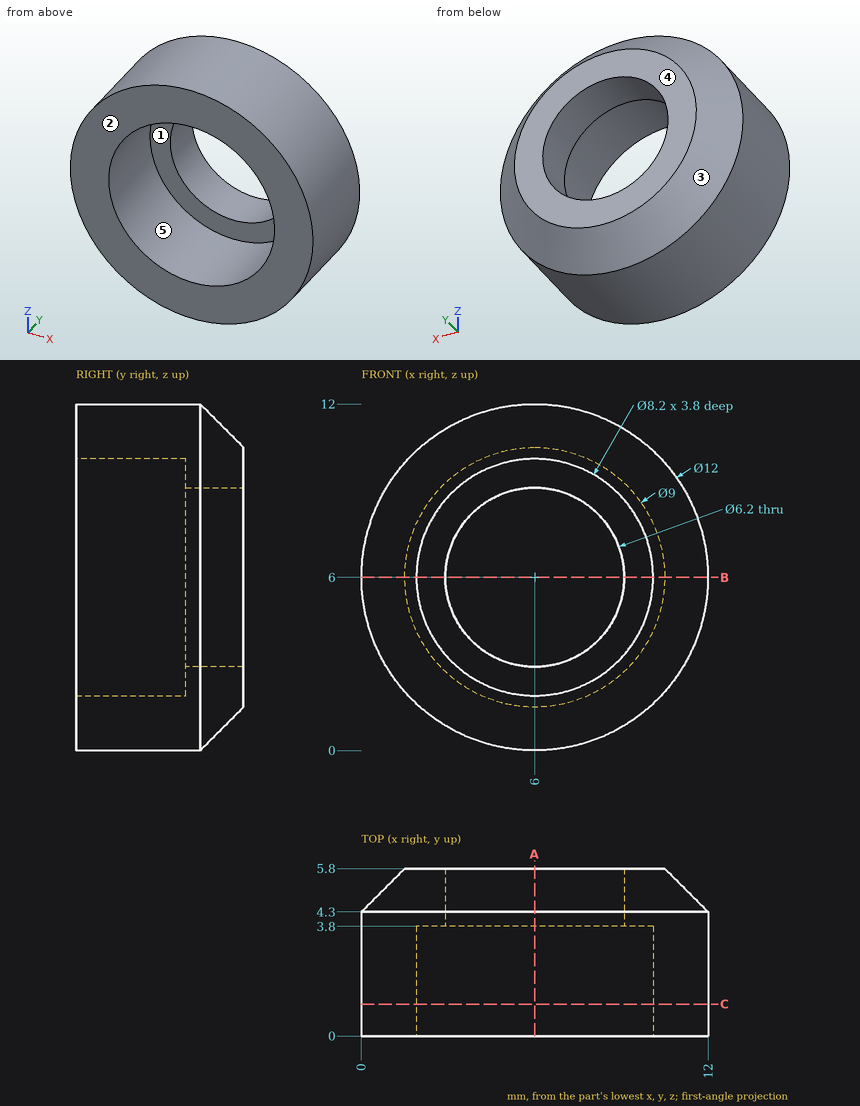
The drawing under review shows one solid part. Ordinate dimensions are in mm from its lowest x, y, z. A direction names the side the tool comes from. Round coordinates to 2 decimals unless told otherwise and drop trailing zeros. Order: outer loops, then holes, each group sorted by start corner. A loop starts at its lowest first (then second) coordinate and runs counter-clockwise, first axis right, second up. Notation, with made-up numbers: (80, 54.5) -> (129, 54.5) arc R4 cw to (129, 59.5) -> close; hole circle Ø5 at (46.25, 69.25). An arc over 180 degrees is marked (long way). Return JSON: item names as keys, results as strings.
1. The part is to be moulded in two halves that separate along Z. For the marked faces 3, 4 and 5, say which applies: +Z half, -Z half, draft (parallel to the pull), parting line (faces both ways), or undercut.
Answer block:
{"face 3": "parting line", "face 4": "draft", "face 5": "undercut"}
2. Take a section at C-C (y = 1.1). Write out the cut boundary in (x, z).
Answer block:
{"outline": "circle Ø12 at (6, 6); hole circle Ø8.2 at (6, 6)"}
3. For the marked faces 1 and 2, list the 3-axis set-ups (+Z, -Z, +X, -X, +Y, -Y) from which the entire face can be reached by the end or side of a thin tool; tool diameter is ignored.
Answer block:
{"face 1": "-Y", "face 2": "+Z, -Z, +X, -X, -Y"}
4. Take a section at A-A (x = 6). Write out the cut boundary in (y, z).
Answer block:
{"outline": "(0, 0) -> (4.3, 0) -> (5.8, 1.5) -> (5.8, 2.9) -> (3.8, 2.9) -> (3.8, 1.9) -> (0, 1.9) -> close; (0, 10.1) -> (3.8, 10.1) -> (3.8, 9.1) -> (5.8, 9.1) -> (5.8, 10.5) -> (4.3, 12) -> (0, 12) -> close"}
5. For L1, parallel to X at y = 1.4, z = 6; L2, parallel to Z at x = 2.5, y = 2.85; L3, parallel to X at y = 2.05, z = 3, list the stretches that pass through material, from the lowest coordinate up. Write a range as [from, to].
Answer block:
{"L1": "x = [0, 1.9], [10.1, 12]", "L2": "z = [1.13, 3.86], [8.14, 10.87]", "L3": "x = [0.8, 3.21], [8.79, 11.2]"}
6. Take a section at B-B (z = 6). Write out the cut boundary in (x, y).
Answer block:
{"outline": "(0, 0) -> (1.9, 0) -> (1.9, 3.8) -> (2.9, 3.8) -> (2.9, 5.8) -> (1.5, 5.8) -> (0, 4.3) -> close; (9.1, 3.8) -> (10.1, 3.8) -> (10.1, 0) -> (12, 0) -> (12, 4.3) -> (10.5, 5.8) -> (9.1, 5.8) -> close"}
7. Insertion check: P1, Ø1, axis at y = 2.5, z = 9, coming from the -X side; P2, Ø2.5, axis at x = 7.5, z = 8, coming from the -Y side; P3, Ø2, axis at x = 3, z = 8, coming from the -Y side. Each pin has a flat end and moves straight along its axis. Give the tip position at first contact, or say it passes through.
Answer block:
{"P1": "stops at x = 0.55", "P2": "stops at y = 3.8", "P3": "stops at y = 0"}
